from build123d import *

# Parameters (mm, degrees)
F0_R      = 112.6860587027
F1_DEPTH  = 101.6
F2_R      = 105.9744016923
F3_DEPTH  = 88.9
F4_DEPTH  = 25.4
F5_DEPTH  = 25.4
F6_W      = 9.2725791037
F6_H      = 8.4680765867
F7_DEPTH  = 12.7
F8_R      = 7.6321412637
F9_DEPTH  = 25.4
F10_W     = 4.2340382934
F10_H     = 13.9821412637
F11_DEPTH = 38.1
F12_W     = 4.2340382934
F12_H     = 6.35
F13_DEPTH = 0.762


with BuildPart() as f1:
    # F0 (on Top) → F1 (new body)
    with BuildSketch(Plane.XY):
        Circle(F0_R)
    extrude(amount=F1_DEPTH)

    # F2 (on face) → F3 (cut)
    with BuildSketch(Plane.XY.offset(101.6)):
        Circle(F2_R)
    extrude(amount=-F3_DEPTH, mode=Mode.SUBTRACT)

    # F4 (add): a face of the model
    f4_faces = [f1.faces().sort_by_distance(p)[0] for p in [
        (0, 0, 12.7),
    ]]
    extrude(f4_faces, amount=F4_DEPTH)

    # F5 (add): a face of the model
    f5_faces = [f1.faces().sort_by_distance(p)[0] for p in [
        (0, 0, 38.1),
    ]]
    extrude(f5_faces, amount=F5_DEPTH)

    # F6 (on face) → F7 (join)
    with BuildSketch(Plane.XY.offset(63.5)):
        with Locations((-24.9477978796, 93.518204987)):
            Rectangle(F6_W, F6_H)
    extrude(amount=F7_DEPTH)

    # F8 (on face) → F9 (join)
    with BuildSketch(Plane.YZ.offset(-20.3115083277)):
        with Locations((93.518204987, 69.85)):
            Circle(F8_R)
    extrude(amount=F9_DEPTH)

    # F10 (on face) → F11 (join)
    with BuildSketch(Plane.YZ.offset(5.0884916723)):
        with Locations((95.6352241337, 70.4910706319)):
            Rectangle(F10_W, F10_H)
    extrude(amount=-F11_DEPTH)

    # F12 (on face) → F13 (join)
    with BuildSketch(Plane.YZ.offset(5.0884916723)):
        with Locations((95.6352241337, 73.025)):
            Rectangle(F12_W, F12_H)
    extrude(amount=F13_DEPTH)


solid = f1.part
Geometry: final body of the model. Coordinates: model frame, mm. A direction names the side the tool comes from. Round coordinates to 2 decimals unless told otherwise and drop trailing zeros. Loops run counter-clockwise (first coordinate to the right, second up) from the corner with the lowest first, then second, coordinate; pieces in that order, holes last. Notation, with made-up numbers: M 83.5,-3.5 L 89.5,-3.5 A26 cw 89.5,16.5 Z; hole C 82,-25 d4. An arc over 180 degrees is marked long. Put each result on its own line as item: value. Start each with the question number.
(1) Material intervals for line 1 along Y through (x, z) = (0, 88); line 2 along Y through (x, z) = (0, 72); line 3 along Z through (x, y) = (-24, -48), sorted ascending. Write a range as [from, to].
(2) Section query B-B (y = 0). Return loops of the section in (x, z), then the cut area to 3 significant figures.
(3) Section query C-C (z = 86.5). Return loops of the section in (x, y).
(4) Draft query along Y for faces 1 (the face through (-30, 93.518, 71)), 2 (the face through (107.48, 33.85, 50.09)), 3 (the face through (5.088, 93, 71)), 4 (the face through (-2, 2, 0)). Return one class per face: +Y half, -Y half, draft (parallel to the pull), parting line (faces both ways), or undercut.
(5) Set-up query: faces 5 (the face through (82.9, -66.3, 101.6)), 6 (the face through (-25, 89.284, 70)), 7 (the face through (-7.789, 86.254, 72.192)). Return all of +Z, -Z, +X, -X, +Y, -Y with unobstructed straight access to the full face (end or side cutting, diameter ignored); none if empty.
(6) Contact query for flat-ended pins moving along their axis: pin 1 Ø3.5 at (y, z) = (99.5, 70) entering from -X; pin 2 Ø10 at (x, y) = (-0.5, -30.5) entering from +Z; pin 3 Ø6 at (x, z) = (26, 46.5) entering from -Y. Output: stop coordinate, or through.
(7) Section query D-D (z = 9). Return loops of the section in (x, y).
(8) Section query A-A (x = 0). Return loops of the section in (y, z).
Findings below:
1. line 1: y = [-112.69, -105.97], [105.97, 112.69]
1. line 2: y = [-112.69, -105.97], [86.2, 100.84], [105.97, 112.69]
1. line 3: z = [0, 63.5]
2. outline: M -112.69,0 L 112.69,0 L 112.69,101.6 L 105.97,101.6 L 105.97,63.5 L -105.97,63.5 L -105.97,101.6 L -112.69,101.6 Z
2. area: 14,800 mm2
3. outline: C 0,0 d225.37; hole C 0,0 d211.95
4. face 1: undercut
4. face 2: parting line
4. face 3: undercut
4. face 4: draft
5. face 5: +Z, +X, -X, +Y, -Y
5. face 6: +Z
5. face 7: none
6. pin 1: stops at x = -56.06
6. pin 2: stops at z = 63.5
6. pin 3: stops at y = -110.31
7. outline: C 0,0 d225.37
8. outline: M -112.69,0 L 112.69,0 L 112.69,101.6 L 105.97,101.6 L 105.97,63.5 L 97.75,63.5 A7.63 ccw 97.75,76.2 L 97.75,77.48 L 93.52,77.48 A7.63 ccw 89.28,63.5 L -105.97,63.5 L -105.97,101.6 L -112.69,101.6 Z
